from build123d import *
from build123d import SkipClean  # not in build123d's __all__

# Parameters (mm, degrees)
F1_DEPTH = 25
F3_DEPTH = 5


with BuildPart() as f1:
    # F0 (on Front) → F1 (new body, symmetric)
    with BuildSketch(Plane.XZ):
        with BuildLine():
            Line((0, 27.6668258011), (0, 18.9514327794))
            ThreePointArc((0, 18.9514327794), (18.9514327794, 0), (0, -18.9514327794))
            Line((0, -18.9514327794), (0, -27.6668258011))
            ThreePointArc((0, -27.6668258011), (27.6668258011, 0), (0, 27.6668258011))
        make_face()
    extrude(amount=F1_DEPTH, both=True)

    # F2 (on Front) → F3 (join, symmetric)
    with BuildSketch(Plane.XZ):
        with BuildLine():
            Line((0, 42.4246681583), (0, 27.4246681583))
            ThreePointArc((0, 27.4246681583), (27.4246681583, 0), (0, -27.4246681583))
            Line((0, -27.4246681583), (0, -42.4246681583))
            Line((0, -42.4246681583), (65, -42.4246681583))
            Line((65, -42.4246681583), (65, 42.4246681583))
            Line((65, 42.4246681583), (0, 42.4246681583))
        make_face()
    extrude(amount=F3_DEPTH, both=True)

    # F4: F1 across face


with BuildPart() as f1_1:
    add(f1.part, clean=False)
    with SkipClean():  # cleaning this boolean's faces spoils the solid; the shape is the same uncleaned
        add(f1.part.mirror(Plane(origin=(0, 0, 26.2783197478), x_dir=(0, -1, 0), z_dir=(-1, 0, 0))), clean=False)


solid = f1_1.part
Work out the finished part from the listing and answer in its coordinate system (mm). Give positions to 0.01 mm unless a question says otherwise; leave off trailing zeros. Order: outer loops, then holes, each group sorted by start corner. A loop starts at its lowest first (then second) coordinate and runs counter-clockwise, first axis right, second up. Notation, with made-up numbers: (-37, 27.5) - (9, 27.5) arc R11 ccw to (9, 41.5) - close; hole circle Ø5 at (77, 24.25). An arc over 180 degrees is marked (long way). Answer as CSV lines item,"result". Start each with the question number.
Q1. The part is cut by section B-B (x = -1.5). Write down the section's boundary in (y, z).
Q2. The part is cut by section A-A (z = 0). Write down the section's boundary in (x, y).
Q3. Given pin 1 Ø10 at (x, z) = (44, 28.5) entering from -Y; pin 2 Ø8 at (x, z) = (14.5, -32.5) entering from +Y; pin 3 Ø1 at (y, z) = (14.5, 1) entering from +X, each flat-ended and moving along its own axis, determine where each tip first touches the part or whether it passes through.
Q4. Find the intervals of material crossed by L1, parallel to Y at x = 55.5, z = -19; L2, parallel to Z at x = -11, y = 17.5; L3, parallel to Z at x = -16, y = -9, in increasing order. Write a range as [from, to].
Q5. The part is cut by section D-D (x = -39.5). Write down the section's boundary in (y, z).
Q6. The part is cut by section C-C (y = -17). Write down the section's boundary in (x, z).
Check result:
1,outline,"(-25, -27.63) - (-5, -27.63) - (-5, -42.42) - (5, -42.42) - (5, -27.63) - (25, -27.63) - (25, -18.89) - (-25, -18.89) - close; (-25, 18.89) - (25, 18.89) - (25, 27.63) - (5, 27.63) - (5, 42.42) - (-5, 42.42) - (-5, 27.63) - (-25, 27.63) - close"
2,outline,"(-65, -5) - (-27.67, -5) - (-27.67, -25) - (-18.95, -25) - (-18.95, 25) - (-27.67, 25) - (-27.67, 5) - (-65, 5) - close; (18.95, -25) - (27.67, -25) - (27.67, -5) - (65, -5) - (65, 5) - (27.67, 5) - (27.67, 25) - (18.95, 25) - close"
3,pin 1,"stops at y = -5"
3,pin 2,"stops at y = 5"
3,pin 3,"stops at x = 27.66"
4,L1,"y = [-5, 5]"
4,L2,"z = [-25.39, -15.43], [15.43, 25.39]"
4,L3,"z = [-22.57, -10.16], [10.16, 22.57]"
5,outline,"(-5, -42.42) - (5, -42.42) - (5, 42.42) - (-5, 42.42) - close"
6,outline,"circle Ø55.33 at (0, 0); hole circle Ø37.9 at (0, 0)"
